```python
from build123d import *

# Parameters (mm, degrees)
SKETCH1_W           = 95
SKETCH1_H           = 140
SKETCH1_R           = 1.75
SKETCH1_R_2         = 2.5
BOSS_EXTRUDE1_DEPTH = 4
FILLET1_R           = 3


with BuildPart() as part:
    # Sketch1 → Boss-Extrude1 (new body)
    with BuildSketch(Plane(origin=(0, 0, 0), x_dir=(1, 0, 0), z_dir=(0, 1, 0))):
        Rectangle(SKETCH1_W, SKETCH1_H)
        with Locations(Location((0, 60, 0), (0, 0, 270))):
            Circle(SKETCH1_R, mode=Mode.SUBTRACT)
        with Locations(Location((0, 25, 0), (0, 0, 270))):
            Circle(SKETCH1_R, mode=Mode.SUBTRACT)
        with Locations(Location((0, -25, 0), (0, 0, 90))):
            Circle(SKETCH1_R, mode=Mode.SUBTRACT)
        with Locations(Location((0, -60, 0), (0, 0, 90))):
            Circle(SKETCH1_R, mode=Mode.SUBTRACT)
        with Locations(Location((-15, 60, 0), (0, 0, 270))):
            Circle(SKETCH1_R, mode=Mode.SUBTRACT)
        with Locations(Location((-15, 25, 0), (0, 0, 270))):
            Circle(SKETCH1_R, mode=Mode.SUBTRACT)
        with Locations(Location((-15, -25, 0), (0, 0, 90))):
            Circle(SKETCH1_R, mode=Mode.SUBTRACT)
        with Locations(Location((-15, -60, 0), (0, 0, 90))):
            Circle(SKETCH1_R, mode=Mode.SUBTRACT)
        with Locations(Location((23.75, 0, 0), (0, 0, 270))):
            Circle(SKETCH1_R_2, mode=Mode.SUBTRACT)
    extrude(amount=BOSS_EXTRUDE1_DEPTH)

    # Fillet1
    fillet1_edges = [part.edges().sort_by_distance(p)[0] for p in [
        (47.5, 2, 70),
        (-47.5, 2, 70),
        (-47.5, 2, -70),
        (47.5, 2, -70),
    ]]
    fillet(fillet1_edges, radius=FILLET1_R)


solid = part.part
```
Geometry: final body of the model. Coordinates: model frame, mm. Coordinates: 2 decimals unless noted, no trailing zeros. Loops run counter-clockwise (first coordinate to the right, second up) from the corner with the lowest first, then second, coordinate; pieces in that order, holes last. Notation, with made-up numbers: M 40,9.5 L 75,9.5 A14 cw 75,15.5 Z; hole C 46,77 d4. An arc over 180 degrees is marked long. Put each result on its own line as item: value.
(1) Cut plane D-D on z = 25. Return the cut outline in (x, y).
Answer sheet:
outline: M -47.5,0 L -16.75,0 L -16.75,4 L -47.5,4 Z; M -13.25,0 L -1.75,0 L -1.75,4 L -13.25,4 Z; M 1.75,0 L 47.5,0 L 47.5,4 L 1.75,4 Z
(2) Cut plane B-B on x = 0. Return the cut outline in (y, z).
Answer sheet:
outline: M 0,-70 L 4,-70 L 4,-61.75 L 0,-61.75 Z; M 0,-58.25 L 4,-58.25 L 4,-26.75 L 0,-26.75 Z; M 0,-23.25 L 4,-23.25 L 4,23.25 L 0,23.25 Z; M 0,26.75 L 4,26.75 L 4,58.25 L 0,58.25 Z; M 0,61.75 L 4,61.75 L 4,70 L 0,70 Z
(3) Material intervals for probe 1 along X at (y, z) = (2.55, -25); probe 2 along X at (y, z) = (1.65, 0), sorted ascending.
Answer sheet:
probe 1: x = -47.5 to -16.75, -13.25 to -1.75, 1.75 to 47.5
probe 2: x = -47.5 to 21.25, 26.25 to 47.5
(4) Draft query along X for faces 1 (the face through (-46.64, 2.03, -69.1)), 2 (the face through (46.6, 2.03, -69.14)), 3 (the face through (-1, 4, -1)), 4 (the face through (-0.08, 1.97, 26.75)). Return one class per face: pulls with the +X half, pulls with the -X half, needs draft (parallel to the pull), parting line crosses it, or undercut.
Answer sheet:
face 1: pulls with the -X half
face 2: pulls with the +X half
face 3: needs draft
face 4: undercut
(5) First-contact query: pin 1 (4 mm diameter, centred on x = 0, z = 25, fed in from -Y); pin 2 (2 mm diameter, centred on x = -15, z = -25, fed in from +Y). Flat tips, straight axial feed; report the tip coordinate or a pass-through.
Answer sheet:
pin 1: stops at y = 0
pin 2: passes through
(6) Cut plane C-C on z = 0. Return the cut outline in (x, y).
Answer sheet:
outline: M -47.5,0 L 21.25,0 L 21.25,4 L -47.5,4 Z; M 26.25,0 L 47.5,0 L 47.5,4 L 26.25,4 Z
(7) Cut plane A-A on x = 23.75. Return the cut outline in (y, z), then the cut area to 3 significant figures.
Answer sheet:
outline: M 0,-70 L 4,-70 L 4,-2.5 L 0,-2.5 Z; M 0,2.5 L 4,2.5 L 4,70 L 0,70 Z
area: 540 mm^2
